The listing builds one solid part. Answer for the finished solid, in the listing's coordinates (mm). A direction names the side the tool comes from. Coordinates: 2 decimals unless noted, no trailing zeros. Loops run counter-clockwise (first coordinate to the right, second up) from the corner with the lowest first, then second, coordinate; pieces in that order, holes last. Notation, with made-up numbers: (47, 14) - (73, 14) arc R24 ccw to (73, 52) - close; hole circle Ø2 at (55, 15). An arc over 180 degrees is marked (long way). Write each question's results on one line, items separated by ' | '. Start each with the question number.
(1) Find section C-C on y = 23.1. Determine the outline of the cut face in (x, z), then the cut area to 3 significant figures.
(2) For faces 1 (the flat face through (49.8, 0, 2)), 2 (the flat face through (-49.8, 0, 2)), 3 (the flat face through (-1, -26.8, 2)), 4 (the cylindrical face through (5.12, -3.12, 4.94)), determine the directions among +Z, -Z, +X, -X, +Y, -Y from which every point of the face is accessible in a straight line to the end or side of a thin tool.
(3) Given pin 1 Ø1.6 at (y, z) = (1.5, 2) entering from +X; pin 2 Ø1 at (x, z) = (-24.5, 2) entering from +Y; pin 3 Ø1.6 at (y, z) = (9.5, 2) entering from -X, each flat-ended and moving along its own axis, determine where each tip first touches the part or whether it passes through.
(4) Find section A-A on x = -46.1. Determine the outline of the cut face in (y, z).
(5) Find section B-B on z = 6. Determine the outline of the cut face in (x, y), then the cut area to 3 significant figures.
(6) Consider line 1 (X direction, y = 14.5, z = 1.75); line 2 (Y direction, x = -46, z = 2); line 3 (Y direction, x = 20, z = 1.5). Determine where each line is inside the solid, lowest interval first. Write a range as from..to.
(7) Find section D-D on x = -4. Determine the outline of the cut face in (y, z), then the cut area to 3 significant figures.
(8) Determine the mould class of faces 5 (the cylindrical face through (-45.03, 22.12, 4.94)), 6 (the flat face through (-1, 26.8, 2)), 7 (the flat face through (0, 26, 3)) for opening direction Y: released by +Y, released by -Y, zero draft, split by the parting line, or undercut.
from build123d import *

# Parameters (mm, degrees)
SKETCH1_W        = 102
SKETCH1_H        = 56
PANEL_DEPTH      = 1
SKETCH2_W        = 99.6
SKETCH2_H        = 53.6
SKETCH2_W_2      = 97.2
SKETCH2_H_2      = 51.2
MOUNTS_DEPTH     = 2
SKETCH3_R        = 1.45
ESP_MOUNTS_DEPTH = 8


with BuildPart() as part:
    # Sketch1 → PANEL (new body)
    with BuildSketch(Plane.XY):
        Rectangle(SKETCH1_W, SKETCH1_H)
    extrude(amount=PANEL_DEPTH)

    # Sketch2 → MOUNTS (add)
    with BuildSketch(Plane.XY.offset(1)):
        Rectangle(SKETCH2_W, SKETCH2_H)
        Rectangle(SKETCH2_W_2, SKETCH2_H_2, mode=Mode.SUBTRACT)
    extrude(amount=MOUNTS_DEPTH)

    # Sketch3 → ESP_MOUNTS (add)
    with BuildSketch(Plane.XY.offset(1)):
        with Locations(Location((-46.1, 23.1, 0), (0, 0, 180))):
            Circle(SKETCH3_R)
        with Locations(Location((-46.1, -1.9, 0), (0, 0, 180))):
            Circle(SKETCH3_R)
        with Locations(Location((5.9, 23.1, 0), (0, 0, 180))):
            Circle(SKETCH3_R)
        with Locations(Location((5.9, -1.9, 0), (0, 0, 180))):
            Circle(SKETCH3_R)
    extrude(amount=ESP_MOUNTS_DEPTH)


solid = part.part
Values:
1) outline: (-51, 0) - (51, 0) - (51, 1) - (49.8, 1) - (49.8, 3) - (48.6, 3) - (48.6, 1) - (7.35, 1) - (7.35, 9) - (4.45, 9) - (4.45, 1) - (-44.65, 1) - (-44.65, 9) - (-47.55, 9) - (-47.55, 1) - (-48.6, 1) - (-48.6, 3) - (-49.8, 3) - (-49.8, 1) - (-51, 1) - close | area: 153 mm²
2) face 1: +Z, +X, +Y, -Y | face 2: +Z, -X, +Y, -Y | face 3: +Z, +X, -X, -Y | face 4: +Z
3) pin 1: stops at x = 49.8 | pin 2: stops at y = 26.8 | pin 3: stops at x = -49.8
4) outline: (-28, 0) - (28, 0) - (28, 1) - (26.8, 1) - (26.8, 3) - (25.6, 3) - (25.6, 1) - (24.55, 1) - (24.55, 9) - (21.65, 9) - (21.65, 1) - (-0.45, 1) - (-0.45, 9) - (-3.35, 9) - (-3.35, 1) - (-25.6, 1) - (-25.6, 3) - (-26.8, 3) - (-26.8, 1) - (-28, 1) - close
5) outline: circle Ø2.9 at (-46.1, -1.9); circle Ø2.9 at (-46.1, 23.1); circle Ø2.9 at (5.9, -1.9); circle Ø2.9 at (5.9, 23.1) | area: 26.4 mm²
6) line 1: x = -49.8..-48.6, 48.6..49.8 | line 2: y = -26.8..-25.6, -3.35..-0.45, 21.65..24.55, 25.6..26.8 | line 3: y = -26.8..-25.6, 25.6..26.8
7) outline: (-28, 0) - (28, 0) - (28, 1) - (26.8, 1) - (26.8, 3) - (25.6, 3) - (25.6, 1) - (-25.6, 1) - (-25.6, 3) - (-26.8, 3) - (-26.8, 1) - (-28, 1) - close | area: 60.8 mm²
8) face 5: undercut | face 6: released by +Y | face 7: zero draft
